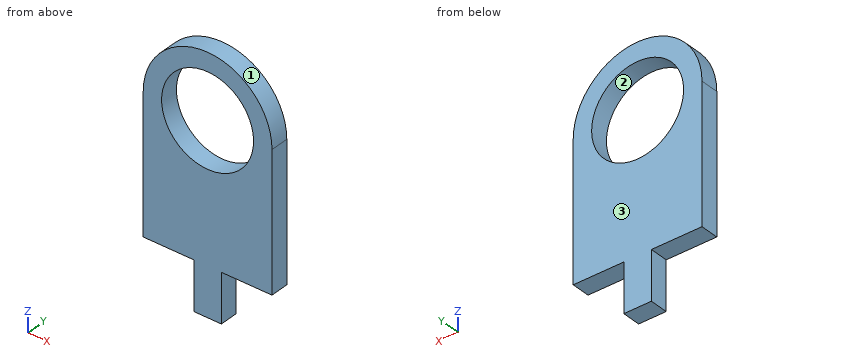
```python
from build123d import *

# Parameters (mm, degrees)
SKETCH1_R           = 25
BOSS_EXTRUDE2_DEPTH = 10


with BuildPart() as part:
    # Sketch1 → Boss-Extrude2 (new body)
    with BuildSketch(Plane(origin=(0, 0, 0), x_dir=(1, 0, 0), z_dir=(0, 1, 0))):
        with BuildLine():
            Line((-35, 74.53460287), (-35, 0))
            ThreePointArc((-35, 0), (0, -35), (35, 0))
            Line((35, 0), (35, 74.53460287))
            Line((35, 74.53460287), (7.5, 74.53460287))
            Line((7.5, 74.53460287), (7.5, 101.011615082))
            Line((7.5, 101.011615082), (-7.5, 101.011615082))
            Line((-7.5, 101.011615082), (-7.5, 74.53460287))
            Line((-7.5, 74.53460287), (-35, 74.53460287))
        make_face()
        Circle(SKETCH1_R, mode=Mode.SUBTRACT)
    extrude(amount=BOSS_EXTRUDE2_DEPTH)


solid = part.part
```
Geometry check sheet. Reference: the model listing, model coordinates, mm. Face numbers are marked on the shaded views. Give positions to 0.01 mm unless a question says otherwise; leave off trailing zeros. Order: outer loops, then holes, each group sorted by start corner. A loop starts at its lowest first (then second) coordinate and runs counter-clockwise, first axis right, second up.
1. Thickness scan on L1, parallel to Z at x = 0, y = 3; L2, parallel to X at y = 6.75, z = -4; L3, parallel to Z at x = 2.5, y = 3.25. Record the ranges inside material, lowest first.
2. Release check for a two-part mould opening along X. For the marked faces 1, 2 and 3 record: pulls with the +X half, pulls with the -X half, needs draft (parallel to the pull), parting line crosses it, or undercut.
3. Gauge pin test, flat ends, axial feed: pin 1 Ø1.5 at (y, z) = (8.5, 20) entering from -X; pin 2 Ø5 at (x, y) = (-16, 4.5) entering from -Z; pin 3 Ø5 at (y, z) = (5, -87.5) entering from -X. Record the tip position at first contact, or that the pin passes through.
4. Section check C-C, the plane z = 1.5. Enter the section's corners in (x, y), and give its area (3 significant figures).
5. Section check D-D, the plane x = 28. Enter the section's corners in (y, z), and give its area (3 significant figures).
6. Section check A-A, the plane y = 2. Enter the section's corners in (x, z).
7. Section check B-B, the plane x = 0. Enter the section's corners in (y, z).
Values follow:
1. L1: z = -101.01 to -25, 25 to 35
1. L2: x = -35 to -24.68, 24.68 to 35
1. L3: z = -101.01 to -24.87, 24.87 to 34.91
2. face 1: parting line crosses it
2. face 2: undercut
2. face 3: needs draft
3. pin 1: stops at x = -29.23
3. pin 2: stops at z = -74.53
3. pin 3: stops at x = -7.5
4. outline: (-34.97, 0) - (-24.95, 0) - (-24.95, 10) - (-34.97, 10) - close; (24.95, 0) - (34.97, 0) - (34.97, 10) - (24.95, 10) - close
4. area: 200 mm2
5. outline: (0, -74.53) - (10, -74.53) - (10, 21) - (0, 21) - close
5. area: 955 mm2
6. outline: (-35, -74.53) - (-7.5, -74.53) - (-7.5, -101.01) - (7.5, -101.01) - (7.5, -74.53) - (35, -74.53) - (35, 0) arc R35 ccw to (-35, 0) - close; hole circle Ø50 at (0, 0)
7. outline: (0, -101.01) - (10, -101.01) - (10, -25) - (0, -25) - close; (0, 25) - (10, 25) - (10, 35) - (0, 35) - close
